```python
from build123d import *

# Parameters (mm, degrees)
SKETCH1_R           = 11
BOSS_EXTRUDE1_DEPTH = 19
SKETCH2_R           = 3.9
BOSS_EXTRUDE2_DEPTH = 9
SKETCH3_R           = 22
SKETCH3_R_2         = 2.75
BOSS_EXTRUDE3_DEPTH = 2.4


with BuildPart() as part:
    # Sketch1 → Boss-Extrude1 (new body)
    with BuildSketch(Plane(origin=(0, 0, 0), x_dir=(1, 0, 0), z_dir=(0, 1, 0))):
        with Locations(Location((0, 0, 0), (0, 0, 270))):
            Circle(SKETCH1_R)
    extrude(amount=BOSS_EXTRUDE1_DEPTH)

    # Sketch2 → Boss-Extrude2 (add)
    with BuildSketch(Plane(origin=(0, 19, 0), x_dir=(1, 0, 0), z_dir=(0, 1, 0))):
        with Locations(Location((0, 0, 0), (0, 0, 270))):
            Circle(SKETCH2_R)
    extrude(amount=BOSS_EXTRUDE2_DEPTH)

    # Sketch3 → Boss-Extrude3 (add)
    with BuildSketch(Plane(origin=(0, 14, 0), x_dir=(1, 0, 0), z_dir=(0, 1, 0))):
        with Locations(Location((0, 0, 0), (0, 0, 270))):
            Circle(SKETCH3_R)
        with Locations(Location((0, -17.5, 0), (0, 0, 270))):
            Circle(SKETCH3_R_2, mode=Mode.SUBTRACT)
        with Locations(Location((-15.155444566, 8.75, 0), (0, 0, 270))):
            Circle(SKETCH3_R_2, mode=Mode.SUBTRACT)
        with Locations(Location((15.155444566, 8.75, 0), (0, 0, 270))):
            Circle(SKETCH3_R_2, mode=Mode.SUBTRACT)
    extrude(amount=-BOSS_EXTRUDE3_DEPTH)


solid = part.part
```
Read the model definition and answer for the solid it produces. Units are mm, in the model's axes. A direction names the side the tool comes from. Give positions to 0.01 mm unless a question says otherwise; leave off trailing zeros. Order: outer loops, then holes, each group sorted by start corner. A loop starts at its lowest first (then second) coordinate and runs counter-clockwise, first axis right, second up.
(1) Find section B-B (z = -9). Give the vertices of the cut face in (x, y), plus the area to 3 significant figures.
(2) For faces 5 (the cylindrical face through (-10.74, 16.46, -2.38)), 6 (the cylindrical face through (-21.477, 12.817, -4.769)), 7 (the cylindrical face through (-10.74, 5.72, -2.38)), determine the directions among +Z, -Z, +X, -X, +Y, -Y from which every point of the face is accessible in a straight line to the end or side of a thin tool.
(3) Straight lines are drawn through the part: L1, parallel to X at y = 13.1, z = -8.75; L2, parallel to Y at x = 20.5, z = 1; L3, parallel to X at y = 12.3, z = 17.5. For each, find the intervals that lie inside material, in ascending order.
(4) Find section C-C (z = 17.5). Give the vertices of the cut face in (x, y).
(5) Find section D-D (z = 0). Give the vertices of the cut face in (x, y), plus the area to 3 significant figures.
(6) Find section A-A (x = 0). Give the vertices of the cut face in (y, z).
(7) For a pull along Z with two mould halves and no side action, classify faces 1 (the cylindrical face through (0.121, 12.817, 14.753)), 2 (the cylindrical face through (-2.373, 23.437, -3.095)), 3 (the cylindrical face through (12.47, 12.82, -9.35)), 4 (the flat face through (0, 28, 0)) as released by +Z, released by -Z, zero draft, split by the parting line, or undercut.
(8) Given pin 1 (3 mm diameter, centred on x = -2, z = 17.5, fed in from +Y); pin 2 (4 mm diameter, centred on y = 12.5, z = 9.5, fed in from -X); pin 3 (5 mm diameter, centred on x = 15.16, z = -8.75, fed in from -Y); pin 4 (12 mm diameter, centred on x = 15.5, z = -0.5, fed in from -Y), each flat-ended and moving along its own axis, determine where each tip first touches the part or whether it passes through.
Result sheet:
1. outline: (-20.07, 11.6) - (-17.89, 11.6) - (-17.89, 14) - (-20.07, 14) - close; (-12.42, 11.6) - (-6.32, 11.6) - (-6.32, 0) - (6.32, 0) - (6.32, 11.6) - (12.42, 11.6) - (12.42, 14) - (6.32, 14) - (6.32, 19) - (-6.32, 19) - (-6.32, 14) - (-12.42, 14) - close; (17.89, 11.6) - (20.07, 11.6) - (20.07, 14) - (17.89, 14) - close
1. area: 280 mm2
2. face 5: +Y
2. face 6: +Y, -Y
2. face 7: -Y
3. L1: x = -20.19 to -17.91, -12.41 to 12.41, 17.91 to 20.19
3. L2: y = 11.6 to 14
3. L3: x = -13.33 to -2.75, 2.75 to 13.33
4. outline: (-13.33, 11.6) - (-2.75, 11.6) - (-2.75, 14) - (-13.33, 14) - close; (2.75, 11.6) - (13.33, 11.6) - (13.33, 14) - (2.75, 14) - close
5. outline: (-22, 11.6) - (-11, 11.6) - (-11, 0) - (11, 0) - (11, 11.6) - (22, 11.6) - (22, 14) - (11, 14) - (11, 19) - (3.9, 19) - (3.9, 28) - (-3.9, 28) - (-3.9, 19) - (-11, 19) - (-11, 14) - (-22, 14) - close
5. area: 541 mm2
6. outline: (0, -11) - (11.6, -11) - (11.6, -22) - (14, -22) - (14, -11) - (19, -11) - (19, -3.9) - (28, -3.9) - (28, 3.9) - (19, 3.9) - (19, 11) - (14, 11) - (14, 14.75) - (11.6, 14.75) - (11.6, 11) - (0, 11) - close; (11.6, 20.25) - (14, 20.25) - (14, 22) - (11.6, 22) - close
7. face 1: undercut
7. face 2: split by the parting line
7. face 3: undercut
7. face 4: zero draft
8. pin 1: stops at y = 14
8. pin 2: stops at x = -20.68
8. pin 3: passes through
8. pin 4: stops at y = 0
